from build123d import *

# Parameters (mm, degrees)
SKETCH2_R               = 4.15
BOSS_EXTRUDE1_DEPTH     = 18
SKETCH3_R               = 1.75
CUT_EXTRUDE1_DEPTH      = 10
CUT_EXTRUDE2_DEPTH      = 19.932643767
CUT_EXTRUDE2_DEPTH_BACK = 19.932643767
SKETCH4_R               = 1.5
FILLET1_R               = 2


with BuildPart() as part:
    # Sketch2 → Boss-Extrude1 (new body)
    with BuildSketch(Plane(origin=(0, 0, 0), x_dir=(1, 0, 0), z_dir=(0, 1, 0))):
        with Locations(Location((0, 0, 0), (0, 0, 270))):
            Circle(SKETCH2_R)
    extrude(amount=BOSS_EXTRUDE1_DEPTH)

    # Sketch3 → Cut-Extrude1 (cut)
    with BuildSketch(Plane.XZ):
        with Locations(Location((0, 0, 0), (0, 0, 270))):
            Circle(SKETCH3_R)
    extrude(amount=-CUT_EXTRUDE1_DEPTH, mode=Mode.SUBTRACT)

    # Sketch4 → Cut-Extrude2 (cut, two sides: drawn at the far end of the back side and taken through both)
    with BuildSketch(Plane(origin=(0, 0, 0), x_dir=(0, 0, -1), z_dir=(1, 0, 0)).offset(-CUT_EXTRUDE2_DEPTH_BACK)):
        with Locations((0, 14)):
            Circle(SKETCH4_R)
    extrude(amount=CUT_EXTRUDE2_DEPTH + CUT_EXTRUDE2_DEPTH_BACK, mode=Mode.SUBTRACT)

    # Fillet1
    fillet1_edges = [part.edges().sort_by_distance(p)[0] for p in [
        (0, 18, -4.15),
    ]]
    fillet(fillet1_edges, radius=FILLET1_R)


solid = part.part
Verification items for the finished model (mm, model axes). A direction names the side the tool comes from. Give positions to 0.01 mm unless a question says otherwise; leave off trailing zeros. Order: outer loops, then holes, each group sorted by start corner. A loop starts at its lowest first (then second) coordinate and runs counter-clockwise, first axis right, second up. Notation, with made-up numbers: M 52.25,46.5 L 76.25,46.5 A28 ccw 76.25,65.5 Z; hole C -21,27 d10. An arc over 180 degrees is marked long. Answer as a JSON object with one key per item and string values. Group by question number.
1) Access from +Z, -Z, +X, -X, +Y, -Y to the whole of each face (thin tool, end or side, straight path). Record for faces 4 (the face through (-1.71, 4.93, 0.38)), 5 (the face through (-0.058, 12.536, 0.325)).
2) Depth check by flat-ended pin: pin 1 Ø1 at (x, z) = (-0.5, -0.5) entering from -Y; pin 2 Ø3 at (x, y) = (-2.5, 2) entering from -Z; pin 3 Ø1 at (x, y) = (-1.5, 6.5) entering from +Z; pin 4 Ø3.5 at (y, z) = (14, 0) entering from -X. Enter the tip coordinate at first touch or a pass-through.
3) Cross-section at B-B (z = 0). Enter the section's corners in (x, y).
4) Cross-section at A-A (x = 0). Enter the section's corners in (y, z), then the cut area to 3 significant figures.
5) Mould release check, pull along X, two halves, no side actions. Record for faces 1 (the face through (0, 10, 0)), 2 (the face through (0, 0, 2)), 3 (the face through (-1.589, 7.888, 3.834)): released by +X, released by -X, zero draft, split by the parting line, or undercut.
6) Cross-section at D-D (y = 13.25). Enter the section's corners in (x, z), then the cut area to 3 significant figures.
7) Cross-section at C-C (y = 10.25). Enter the section's corners in (x, z), then the cut area to 3 significant figures.
8) Scan lines: line 1 along X through (y, z) = (7.75, 0); line 2 along Y through (x, z) = (1.5, 0); line 3 along Y through (x, z) = (2, 0). Record each from-to range of solid material in increasing order. Write a range as [from, to].
Result sheet:
{
 "1": {"face 4": "-Y", "face 5": "+X, -X"},
 "2": {"pin 1": "stops at y = 10", "pin 2": "stops at z = -4.03", "pin 3": "stops at z = 4.03", "pin 4": "stops at x = -4.15"},
 "3": {"outline": "M -4.15,0 L -1.75,0 L -1.75,10 L 1.75,10 L 1.75,0 L 4.15,0 L 4.15,12.5 L -4.15,12.5 Z; M -4.15,15.5 L 4.15,15.5 L 4.15,16 A2 ccw 2.15,18 L -2.15,18 A2 ccw -4.15,16 Z"},
 "4": {"outline": "M 0,-4.15 L 16,-4.15 A2 ccw 18,-2.15 L 18,2.15 A2 ccw 16,4.15 L 0,4.15 L 0,1.75 L 10,1.75 L 10,-1.75 L 0,-1.75 Z; hole C 14,0 d3", "area": "106 mm2"},
 "5": {"face 1": "undercut", "face 2": "zero draft", "face 3": "split by the parting line"},
 "6": {"outline": "M -3.94,-1.3 A4.15 ccw 3.94,-1.3 Z; M -3.94,1.3 L 3.94,1.3 A4.15 ccw Z", "area": "32.9 mm2"},
 "7": {"outline": "C 0,0 d8.3", "area": "54.1 mm2"},
 "8": {"line 1": "x = [-4.15, -1.75], [1.75, 4.15]", "line 2": "y = [10, 12.5], [15.5, 18]", "line 3": "y = [0, 12.5], [15.5, 18]"}
}
